CAD build for the part. Positions are in the model's coordinates, mm. A direction names the side the tool comes from. Coordinates: 2 decimals unless noted, no trailing zeros. Write item = value, one per line. Start each with the question number.
```python
from build123d import *

# Parameters (mm, degrees)
BOSS_EXTRUDE1_DEPTH = 45
FILLET1_R           = 7
FILLET3_R           = 3
FILLET4_R           = 3
FILLET5_R           = 2
FILLET6_R           = 0.5


with BuildPart() as part:
    # Sketch1 → Boss-Extrude1 (new, symmetric)
    with BuildSketch(Plane(origin=(0, 0, 0), x_dir=(0, 0, -1), z_dir=(1, 0, 0))):
        Polygon((-20.062717328, 29.958093621), (-27.716385975, 11.480502971), (0, 0), (21.04758878, 50.813374288), (31.04758878, 50.813374288), (53.62591129, -3.69551813), (54.259961961, -5.22625186), (49.93039316, -5.22625186), (28.374874228, 46.813374288), (23.720303332, 46.813374288), (2.164784401, -5.22625186), (-32.942637835, 9.31571857), (-23.758235458, 31.488827351), align=None)
    extrude(amount=BOSS_EXTRUDE1_DEPTH, both=True)

    # Fillet1
    fillet1_edges = [part.edges().sort_by_distance(p)[0] for p in [
        (0, 50.813374288, -21.04758878),
        (0, 50.813374288, -31.04758878),
    ]]
    fillet(fillet1_edges, radius=FILLET1_R)

    # Fillet3
    fillet3_edges = [part.edges().sort_by_distance(p)[0] for p in [
        (0, 46.813374288, -28.374874228),
        (0, 46.813374288, -23.720303332),
    ]]
    fillet(fillet3_edges, radius=FILLET3_R)

    # Fillet4
    fillet4_edges = [part.edges().sort_by_distance(p)[0] for p in [
        (0, -5.22625186, -2.164784401),
        (0, 9.31571857, 32.942637835),
    ]]
    fillet(fillet4_edges, radius=FILLET4_R)

    # Fillet5
    fillet5_edges = [part.edges().sort_by_distance(p)[0] for p in [
        (0, 29.958093621, 20.062717328),
        (0, 31.488827351, 23.758235458),
    ]]
    fillet(fillet5_edges, radius=FILLET5_R - 0.0001)  # a hair under: the kernel refuses the full size

    # Fillet6
    fillet6_edges = [part.edges().sort_by_distance(p)[0] for p in [
        (-45, 19.795464958, 24.27221595),
        (-45, 5.740251485, 13.858192988),
        (-45, 20.632953228, -43.548728501),
        (-45, -5.22625186, -52.09517756),
        (45, -5.22625186, -52.09517756),
        (45, 20.632953228, -43.548728501),
        (-45, 23.246079157, -9.628841259),
        (45, 23.246079157, -9.628841259),
        (-45, 50.813374288, -26.04758878),
        (-45, 49.633661574, -30.259329946),
        (-45, 49.633661574, -21.835847614),
        (45, 50.813374288, -26.04758878),
        (45, 49.633661574, -30.259329946),
        (45, 49.633661574, -21.835847614),
        (45, 5.740251485, 13.858192988),
        (-45, 19.867586363, -39.536185036),
        (45, 19.867586363, -39.536185036),
        (-45, 46.813374288, -26.04758878),
        (45, 46.813374288, -26.04758878),
        (45, 19.795464958, 24.27221595),
        (-45, 46.307783125, -28.037049014),
        (45, 46.307783125, -28.037049014),
        (-45, 46.307783125, -24.058128546),
        (45, 46.307783125, -24.058128546),
        (-45, 2.044733355, 15.388926717),
        (45, 2.044733355, 15.388926717),
        (-45, 21.253405662, -13.133017673),
        (-45, -4.078201562, -1.689246397),
        (-45, 9.791256574, 31.794587538),
        (45, 21.253405662, -13.133017673),
        (45, -4.078201562, -1.689246397),
        (45, 9.791256574, 31.794587538),
        (-45, 20.864258921, 28.159075796),
        (-45, 30.723498754, 23.441225974),
        (-45, 29.641084137, 20.828045924),
        (45, 20.864258921, 28.159075796),
        (45, 30.723498754, 23.441225974),
        (45, 29.641084137, 20.828045924),
    ]]
    fillet(fillet6_edges, radius=FILLET6_R)


solid = part.part
```
1. Mould opens along Y. For faces 5 (the cylindrical face through (-0.62, 49.6, -30.31)), 6 (the flat face through (1, -5.226, -52)), 7 (the cylindrical face through (44.86, 5.52, 13.72)), 8 (the flat face through (45, 21, -11)) say: released by +Y, released by -Y, zero draft, split by the parting line, or undercut.
2. Flat gauge pins, fed straight in: pin 1 (10 mm diameter, centred on x = -13, z = 22.5, fed in from -Y); pin 2 (5 mm diameter, centred on x = -11.5, y = 44.5, fed in from +Z); pin 3 (8 mm diameter, centred on x = 0.5, y = 18.5, fed in from +Z). Where does each tip first touch, or does it go through?
3. Probe L1, parallel to Z at x = -14.5, y = 12; L2, parallel to Z at x = -23, y = 18.5; L3, parallel to Y at x = -34.5, z = 1.5. List the from-to ranges inside material, lowest first.
4. Slice it at B-B (y = 18.5). Give the number of separate pieces and of enclosed holes in the cut face, plus the area to 3 significant figures.
5. 3-axis set-ups, long thin cutter, end or side, ignore diameter. For faces 1 (the flat face through (0.623, 22.921, -9.494)), 2 (the flat face through (0.62, 5.82, 14.05)), 3 (the flat face through (0.623, 21.585, -13.271)), 4 (the cylindrical face through (-44.85, 20.976, -12.864)): which of +Z, -Z, +X, -X, +Y, -Y reach the whole face in a straight line?
Calculated:
q1.face_5 = released by +Y
q1.face_6 = released by -Y
q1.face_7 = undercut
q1.face_8 = zero draft
q2.pin_1 = 2.92
q2.pin_2 = -17.4
q2.pin_3 = 30.8
q3.L1 = -47.12 to -42.8, -9.3 to -4.97, 27.5 to 31.83
q3.L2 = -44.43 to -40.1, -11.99 to -7.66, 24.81 to 29.14
q3.L3 = -3.71 to 0.62
q4.separate_pieces = 3
q4.enclosed_holes = 0
q4.area = 1,170 mm²
q5.face_1 = +X, -X, +Y
q5.face_2 = +X, -X
q5.face_3 = +X, -X, -Y
q5.face_4 = -X, -Y
